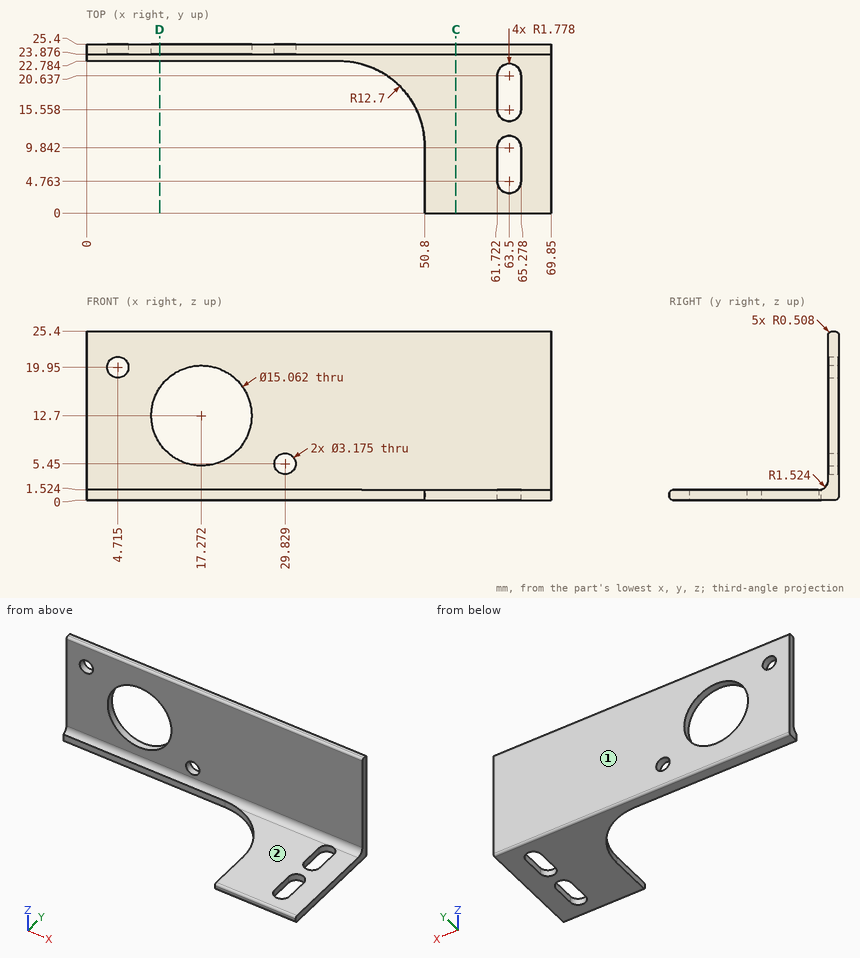
Print and shaded views of the part. All mm, measured from the part's lowest x, y and z. A direction names the side the tool comes from. Give positions to 0.01 mm unless a question says otherwise; leave off trailing zeros. Order: outer loops, then holes, each group sorted by start corner. A loop starts at its lowest first (then second) coordinate and runs counter-clockwise, first axis right, second up. Notation, with made-up numbers: (-10.75, 20) - (45.25, 20) arc R13 ccw to (45.25, 32) - close; hole circle Ø6 at (72.25, 30). An arc over 180 degrees is marked (long way). Use a Markdown table: item, result.
1) 3-axis set-ups, long thin cutter, end or side, ignore diameter. For the marked faces 1 and 2: which of +Z, -Z, +X, -X, +Y, -Y reach the whole face in a straight line?
Checked values:
| item | result |
|---|---|
| face 1 | +Z, -Z, +X, -X, +Y |
| face 2 | +Z, +X, -X, -Y |
2) Flat gauge pins, fed straight in: P1, Ø5, axis at x = 48, z = 9, coming from the -Y side; P2, Ø1.9, axis at x = 4.71, z = 19.95, coming from the +Y side; P3, Ø1.7, axis at y = 17.5, z = 0.5, coming from the -X side; P4, Ø1.3, axis at x = 11.5, z = 1, coming from the -Y side. Where does each tip first touch, or does it go through?
Checked values:
| item | result |
|---|---|
| P1 | y = 23.88 |
| P2 | through |
| P3 | x = 47.74 |
| P4 | y = 22.78 |
3) Probe L1, parallel to Y at x = 20, z = 24 (1 decimal); L2, parallel to Z at x = 56, y = 12.5 (1 decimal); L3, parallel to Z at x = 41.5, y = 22.75. List the from-to ranges inside material, lowest first. Write a range as from..to.
Checked values:
| item | result |
|---|---|
| L1 | 23.9..25.4 |
| L2 | 0..1.5 |
| L3 | 0..1.58 |
4) Saw through at D-D on x = 11. List the corners of the cut face in (y, z) (1 decimal).
Checked values:
| item | result |
|---|---|
| outline | (22.8, 0) - (24.9, 0) arc R0.5 ccw to (25.4, 0.5) - (25.4, 8.5) - (23.9, 8.5) - (23.9, 3) arc R1.5 cw to (22.8, 1.6) - close; (23.9, 16.9) - (25.4, 16.9) - (25.4, 24.9) arc R0.5 ccw to (24.9, 25.4) - (24.4, 25.4) arc R0.5 ccw to (23.9, 24.9) - close |
5) Saw through at C-C on x = 55.5. List the corners of the cut face in (y, z) (1 decimal).
Checked values:
| item | result |
|---|---|
| outline | (0, 0.5) arc R0.5 ccw to (0.5, 0) - (24.9, 0) arc R0.5 ccw to (25.4, 0.5) - (25.4, 24.9) arc R0.5 ccw to (24.9, 25.4) - (24.4, 25.4) arc R0.5 ccw to (23.9, 24.9) - (23.9, 3) arc R1.5 cw to (22.4, 1.5) - (0.5, 1.5) arc R0.5 ccw to (0, 1) - close |
